Check sheet for the drawn part. Datum: minimum x, y, z corner. Units: mm. Give positions to 0.01 mm unless a question says otherwise; leave off trailing zeros. Order: outer loops, then holes, each group sorted by start corner. A loop starts at its lowest first (then second) coordinate and runs counter-clockwise, first axis right, second up.
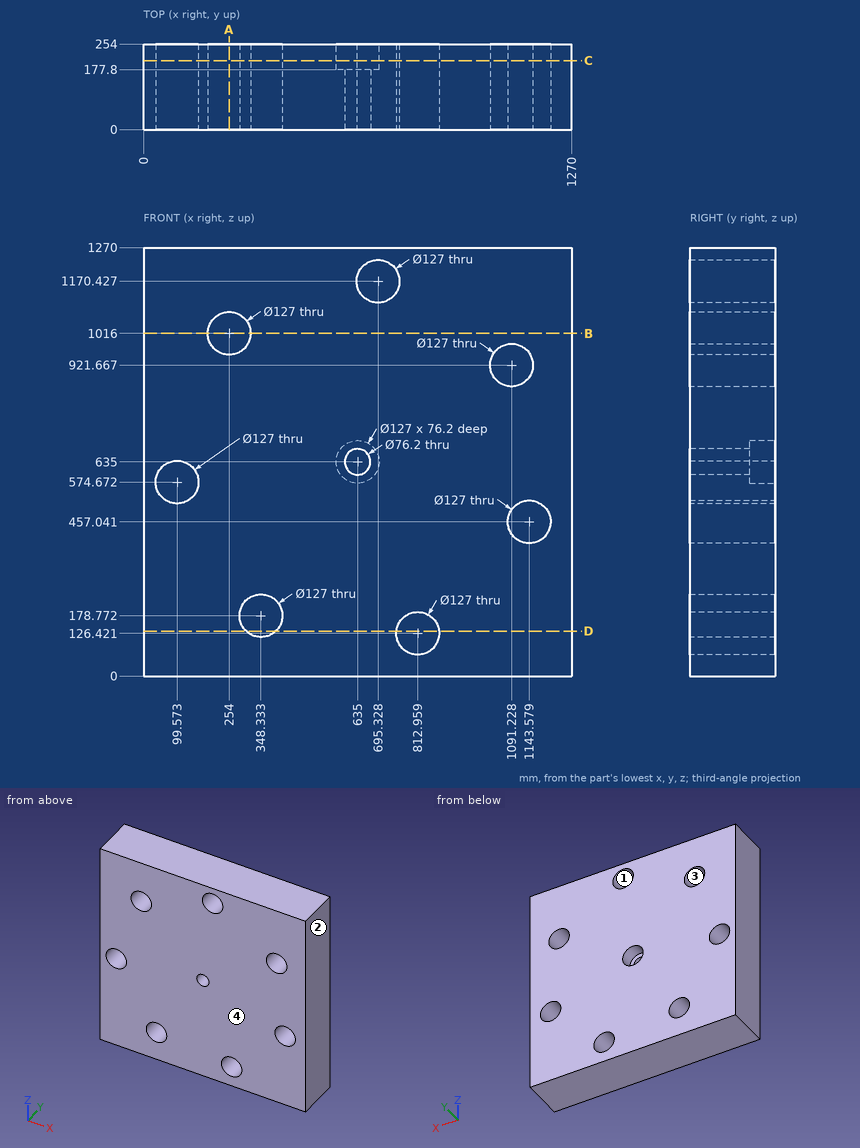
Q1. Sectioned sample at B-B, the plane z = 1016. Record the cut outline in (x, y).
Q2. Sectioned sample at D-D, the plane z = 133. Record the cut outline in (x, y), plus the area to 3 significant figures.
Q3. Material ranges on line 1 (X direction, y = 69.5, z = 460); line 2 (Z direction, x = 1119, y = 159.5); line 3 (X direction, y = 83, z = 1016), recorded low to high.
Q4. Draft check along X on the marked faces 1, 2, 3 and 4. Enter one of: pulls with the +X half, pulls with the -X half, needs draft (parallel to the pull), parting line crosses it, or undercut.
Q5. Sectioned sample at A-A, the plane x = 254. Record the cut outline in (y, z).
Q6. Sectioned sample at C-C, the plane y = 205. Count the separate pieces of the cut face and the enclosed holes in it, plus the area to 3 significant figures.
Filled in:
1. outline: (0, 0) - (190.5, 0) - (190.5, 254) - (0, 254) - close; (317.5, 0) - (1270, 0) - (1270, 254) - (317.5, 254) - close
2. outline: (0, 0) - (304.32, 0) - (304.32, 254) - (0, 254) - close; (392.35, 0) - (749.8, 0) - (749.8, 254) - (392.35, 254) - close; (876.12, 0) - (1270, 0) - (1270, 254) - (876.12, 254) - close
2. area: 268,000 mm2
3. line 1: x = 0 to 1080.15, 1207.01 to 1270
3. line 2: z = 0 to 398.49, 515.59 to 864.56, 978.77 to 1270
3. line 3: x = 0 to 190.5, 317.5 to 1270
4. face 1: undercut
4. face 2: pulls with the +X half
4. face 3: undercut
4. face 4: needs draft
5. outline: (0, 0) - (254, 0) - (254, 952.5) - (0, 952.5) - close; (0, 1079.5) - (254, 1079.5) - (254, 1270) - (0, 1270) - close
6. separate pieces: 1
6. enclosed holes: 8
6. area: 1,510,000 mm2
